```python
from build123d import *

# Parameters (mm, degrees)
SKETCH1_R                       = 12.5
F_25MM_DIA_DEPTH                = 10
F_15MM_START                    = -10
SKETCH2_R                       = 7.5
F_15MM_DIA_BEARING_END_DEPTH    = 40
F_15MM_START_2                  = 55
SKETCH3_R                       = 7.5
F_15MM_DIA_GEAR_END_DEPTH       = 55
M3X0_5_TAPPED_HOLE1_D           = 2.5
M3X0_5_TAPPED_HOLE1_DEPTH       = 15
M3X0_5_TAPPED_HOLE1_CSINK_D     = 4
M3X0_5_TAPPED_HOLE1_CSINK_ANGLE = 120
M3X0_5_TAPPED_HOLE1_TIP         = 0.751075774
CUT_EXTRUDE1_DEPTH              = 2


# Read off the part's stored shape, not the designer's step: M10x1.5 Machine Threads Stud1
with BuildPart() as part:
    # Sketch1 → 25mm dia (new body)
    with BuildSketch(Plane.XY):
        Circle(SKETCH1_R)
    extrude(amount=F_25MM_DIA_DEPTH)

    # Sketch2 → 15mm dia bearing end (add)
    with BuildSketch(Plane.XY.offset(10).offset(F_15MM_START)):
        Circle(SKETCH2_R)
    extrude(amount=F_15MM_DIA_BEARING_END_DEPTH)

    # Sketch3 → 15mm dia gear end (add)
    with BuildSketch(Plane(origin=(0, 0, 0), x_dir=(-1, 0, 0), z_dir=(0, 0, -1)).offset(F_15MM_START_2)):
        with Locations(Location((0, 0, 0), (0, 0, 180))):
            Circle(SKETCH3_R)
    extrude(amount=-F_15MM_DIA_GEAR_END_DEPTH)

    # M3x0.5 Tapped Hole1
    with Locations(Plane.XY.offset(40)):
        with Locations((0, 0)):
            CounterSinkHole(M3X0_5_TAPPED_HOLE1_D / 2, M3X0_5_TAPPED_HOLE1_CSINK_D / 2, depth=M3X0_5_TAPPED_HOLE1_DEPTH, counter_sink_angle=M3X0_5_TAPPED_HOLE1_CSINK_ANGLE)
            with Locations((0, 0, -(M3X0_5_TAPPED_HOLE1_DEPTH + M3X0_5_TAPPED_HOLE1_TIP / 2))):  # 118° drill point
                Cone(0, M3X0_5_TAPPED_HOLE1_D / 2, M3X0_5_TAPPED_HOLE1_TIP, mode=Mode.SUBTRACT)

    # M10x1.5 Machine Threads Stud1 outline → M10x1.5 Machine Threads Stud1 (revolve, cut)
    with BuildSketch(Plane.XZ):
        Polygon((4.172, -55), (7.5, -55), (7.5, -35), (5, -35), (5, -54.172), align=None)
    revolve(axis=Axis((0, 0, 0), (0, 0, 1)), mode=Mode.SUBTRACT)

    # Sketch15 → Cut-Extrude1 (cut)
    with BuildSketch(Plane.ZY.offset(7.5)):
        with BuildLine():
            Line((-35, 2), (-2, 2))
            ThreePointArc((-2, 2), (0, 0), (-2, -2))
            Line((-2, -2), (-35, -2))
            Line((-35, -2), (-35, 2))
        make_face()
    extrude(amount=-CUT_EXTRUDE1_DEPTH, mode=Mode.SUBTRACT)


solid = part.part
```
Check sheet for the modelled part. Datum: model origin and axes. Units: mm. A direction names the side the tool comes from. Round coordinates to 2 decimals unless told otherwise and drop trailing zeros. Order: outer loops, then holes, each group sorted by start corner. A loop starts at its lowest first (then second) coordinate and runs counter-clockwise, first axis right, second up.
1) Mould release check, pull along Y, two halves, no side actions. Record for faces 1 (the cylindrical face through (-7.493, 0.33, 24.79)), 2 (the flat face through (0, -8, 0)), 3 (the flat face through (-5.5, 0, -17)): +Y half, -Y half, draft (parallel to the pull), parting line (faces both ways), or undercut.
2) Section check B-B (y = 6). Record the boundary of the cut face in (x, z).
3) Section check C-C (x = 10). Record the boundary of the cut face in (y, z), and give its area (3 significant figures).
4) Tool access check on faces 4 (the flat face through (2, -2, 40)), 5 (the flat face through (-6, 2, -19)), 6 (the cylindrical face through (-1.08, -4.88, -44.72)), 7 (the cylindrical face through (0.27, -1.22, 32.18)), 8 (the cylindrical face through (11.923, 3.755, 4.93)). Record the directions out of +Z, -Z, +X, -X, +Y, -Y that give a thin tool (end or side, any length) a straight path to the whole face; none if there is none.
5) Section check A-A (z = -20.5). Record the boundary of the cut face in (x, y).
6) Go/stop test with flat-tipped pins: pin 1 Ø2 at (x, y) = (0, 0) entering from +Z; pin 2 Ø2 at (y, z) = (6, -4) entering from +X; pin 3 Ø2 at (x, z) = (0, -12) entering from +Y. Record where each tip stops, or that it passes through.
7) Scan lines: line 1 (X direction, y = 0, z = 35.5); line 2 (Z direction, x = 1.25, y = -7.25). Record each from-to range of solid material in increasing order.
Result:
1. face 1: parting line
1. face 2: draft
1. face 3: undercut
2. outline: (-10.97, 0) - (-4.5, 0) - (-4.5, -35) - (4.5, -35) - (4.5, 0) - (10.97, 0) - (10.97, 10) - (4.5, 10) - (4.5, 40) - (-4.5, 40) - (-4.5, 10) - (-10.97, 10) - close
3. outline: (-7.5, 0) - (7.5, 0) - (7.5, 10) - (-7.5, 10) - close
3. area: 150 mm2
4. face 4: +Z, +X, -X, +Y, -Y
4. face 5: -Z, -X
4. face 6: -Z
4. face 7: +Z
4. face 8: +Z, -Z
5. outline: (-7.23, -2) arc R7.5 ccw (long way) to (-7.23, 2) - (-5.5, 2) - (-5.5, -2) - close
6. pin 1: stops at z = 24.85
6. pin 2: stops at x = 5.59
6. pin 3: stops at y = 7.5
7. line 1: x = -7.5 to -1.25, 1.25 to 7.5
7. line 2: z = -35 to 40
